For this review, take the finished solid that the model builds, in its own axes (mm). Face numbers are marked on the shaded views. A direction names the side the tool comes from. Coordinates: 2 decimals unless noted, no trailing zeros. Loops run counter-clockwise (first coordinate to the right, second up) from the corner with the lowest first, then second, coordinate; pieces in that order, holes last. Notation, with made-up numbers: (18, 39) -> (33, 39) arc R14 ccw to (33, 61) -> close; hole circle Ø3 at (29.25, 53). An arc over 180 degrees is marked (long way). Use a Markdown table: item, result.
from build123d import *
from build123d.topology import SkipClean

# Parameters (mm, degrees)
SKETCH1_W                 = 57.15
SKETCH1_H                 = 37.592
BOSS_EXTRUDE1_DEPTH       = 10.16
SKETCH2_W                 = 0.254
SKETCH2_H                 = 37.592
SKETCH2_W_2               = 2.032
BOSS_EXTRUDE2_DEPTH       = 2.54
SKETCH3_R                 = 6.35
CUT_EXTRUDE1_DEPTH        = 21.082
SKETCH4_R                 = 2.032
CUT_EXTRUDE2_DEPTH        = 5.08
SKETCH5_W                 = 2.54
SKETCH5_H                 = 0.254
BOSS_EXTRUDE3_DEPTH       = 3.048
MIRROR2_COPY_1_SKETCH_W   = 57.15
MIRROR2_COPY_1_SKETCH_H   = 37.592
MIRROR2_COPY_1_DEPTH      = 10.16
MIRROR2_COPY_2_SKETCH_W   = 0.254
MIRROR2_COPY_2_SKETCH_H   = 37.592
MIRROR2_COPY_2_SKETCH_W_2 = 2.032
MIRROR2_COPY_2_DEPTH      = 2.54
MIRROR2_COPY_3_SKETCH_R   = 6.35
MIRROR2_COPY_3_DEPTH      = 21.082
MIRROR2_COPY_4_SKETCH_R   = 2.032
MIRROR2_COPY_4_DEPTH      = 5.08
MIRROR2_COPY_5_SKETCH_W   = 2.54
MIRROR2_COPY_5_SKETCH_H   = 0.254
MIRROR2_COPY_5_DEPTH      = 3.048


with BuildPart() as part:
    # Sketch1 → Boss-Extrude1 (new body)
    with BuildSketch(Plane.XY):
        with Locations((0.47625, 18.796)):
            Rectangle(SKETCH1_W, SKETCH1_H)
    boss_extrude1 = extrude(amount=BOSS_EXTRUDE1_DEPTH)

    # Sketch2 → Boss-Extrude2 (add)
    with BuildSketch(Plane.XY.offset(10.16)):
        with Locations((-19.97075, 18.796)):
            Rectangle(SKETCH2_W, SKETCH2_H)
        with Locations((-18.57375, 18.796)):
            Rectangle(SKETCH2_W_2, SKETCH2_H)
        with Locations((-17.17675, 18.796)):
            Rectangle(SKETCH2_W, SKETCH2_H)
    boss_extrude2 = extrude(amount=BOSS_EXTRUDE2_DEPTH)

    # Sketch3 → Cut-Extrude1 (cut)
    with BuildSketch(Plane.XY.offset(10.16)):
        with Locations((-28.09875, 0)):
            Circle(SKETCH3_R)
    cut_extrude1 = extrude(amount=-CUT_EXTRUDE1_DEPTH, mode=Mode.SUBTRACT)

    # Sketch4 → Cut-Extrude2 (cut)
    with BuildSketch(Plane(origin=(0, 0, 0), x_dir=(-1, 0, 0), z_dir=(0, 0, -1))):
        with Locations((12.004431959, 16.094318041)):
            Circle(SKETCH4_R)
    cut_extrude2 = extrude(amount=-CUT_EXTRUDE2_DEPTH, mode=Mode.SUBTRACT)

    # Sketch5 → Boss-Extrude3 (add)
    with BuildSketch(Plane.ZY.offset(20.09775)):
        with Locations((11.43, 37.465)):
            Rectangle(SKETCH5_W, SKETCH5_H)
    boss_extrude3 = extrude(amount=-BOSS_EXTRUDE3_DEPTH)

    # Mirror1: Boss-Extrude1, Boss-Extrude2, Cut-Extrude1, Cut-Extrude2, Boss-Extrude3 across plane
    with SkipClean():  # the faces are left unmerged after this step: merging them gives an invalid solid
        add(boss_extrude1.mirror(Plane(origin=(-28.09875, 37.592, 10.16), x_dir=(0, 0, 1), z_dir=(1, 0, 0))))
        add(boss_extrude2.mirror(Plane(origin=(-28.09875, 37.592, 10.16), x_dir=(0, 0, 1), z_dir=(1, 0, 0))))
        add(cut_extrude1.mirror(Plane(origin=(-28.09875, 37.592, 10.16), x_dir=(0, 0, 1), z_dir=(1, 0, 0))), mode=Mode.SUBTRACT)
        add(cut_extrude2.mirror(Plane(origin=(-28.09875, 37.592, 10.16), x_dir=(0, 0, 1), z_dir=(1, 0, 0))), mode=Mode.SUBTRACT)
        add(boss_extrude3.mirror(Plane(origin=(-28.09875, 37.592, 10.16), x_dir=(0, 0, 1), z_dir=(1, 0, 0))))
    add(part.part.scale(1), mode=Mode.REPLACE)  # the faces are merged on a copy

    # Mirror2: Boss-Extrude1, Boss-Extrude2, Cut-Extrude1, Cut-Extrude2, Boss-Extrude3 across plane
    with SkipClean():  # the faces are left unmerged after this step: merging them gives an invalid solid
        add(boss_extrude1.mirror(Plane.ZX))
        add(boss_extrude2.mirror(Plane.ZX))
        add(cut_extrude1.mirror(Plane.ZX), mode=Mode.SUBTRACT)
        add(cut_extrude2.mirror(Plane.ZX), mode=Mode.SUBTRACT)
        add(boss_extrude3.mirror(Plane.ZX))
    add(part.part.scale(1), mode=Mode.REPLACE)  # the faces are merged on a copy

    # Mirror2 copy 1 sketch → Mirror2 copy 1 (add)
    with BuildSketch(Plane(origin=(-56.1975, 0, 0), x_dir=(-1, 0, 0), z_dir=(0, 0, 1))):
        with Locations((0.47625, 18.796)):
            Rectangle(MIRROR2_COPY_1_SKETCH_W, MIRROR2_COPY_1_SKETCH_H)
    extrude(amount=MIRROR2_COPY_1_DEPTH)

    # Mirror2 copy 2 sketch → Mirror2 copy 2 (add)
    with BuildSketch(Plane(origin=(-56.1975, 0, 10.16), x_dir=(-1, 0, 0), z_dir=(0, 0, 1))):
        with Locations((-19.97075, 18.796)):
            Rectangle(MIRROR2_COPY_2_SKETCH_W, MIRROR2_COPY_2_SKETCH_H)
        with Locations((-18.57375, 18.796)):
            Rectangle(MIRROR2_COPY_2_SKETCH_W_2, MIRROR2_COPY_2_SKETCH_H)
        with Locations((-17.17675, 18.796)):
            Rectangle(MIRROR2_COPY_2_SKETCH_W, MIRROR2_COPY_2_SKETCH_H)
    extrude(amount=MIRROR2_COPY_2_DEPTH)

    # Mirror2 copy 3 sketch → Mirror2 copy 3 (cut)
    with SkipClean():  # the faces are left unmerged after this step: merging them gives an invalid solid
        with BuildSketch(Plane(origin=(-56.1975, 0, 10.16), x_dir=(-1, 0, 0), z_dir=(0, 0, 1))):
            with Locations((-28.09875, 0)):
                Circle(MIRROR2_COPY_3_SKETCH_R)
        extrude(amount=-MIRROR2_COPY_3_DEPTH, mode=Mode.SUBTRACT)

    # Mirror2 copy 4 sketch → Mirror2 copy 4 (cut)
    with SkipClean():  # the faces are left unmerged after this step: merging them gives an invalid solid
        with BuildSketch(Plane(origin=(-56.1975, 0, 0), x_dir=(1, 0, 0), z_dir=(0, 0, -1))):
            with Locations((12.004431959, 16.094318041)):
                Circle(MIRROR2_COPY_4_SKETCH_R)
        extrude(amount=-MIRROR2_COPY_4_DEPTH, mode=Mode.SUBTRACT)

    # Mirror2 copy 5 sketch → Mirror2 copy 5 (add)
    with SkipClean():  # the faces are left unmerged after this step: merging them gives an invalid solid
        with BuildSketch(Plane(origin=(-36.09975, 0, 0), x_dir=(0, 0, 1), z_dir=(1, 0, 0))):
            with Locations((11.43, 37.465)):
                Rectangle(MIRROR2_COPY_5_SKETCH_W, MIRROR2_COPY_5_SKETCH_H)
        extrude(amount=-MIRROR2_COPY_5_DEPTH)


solid = part.part
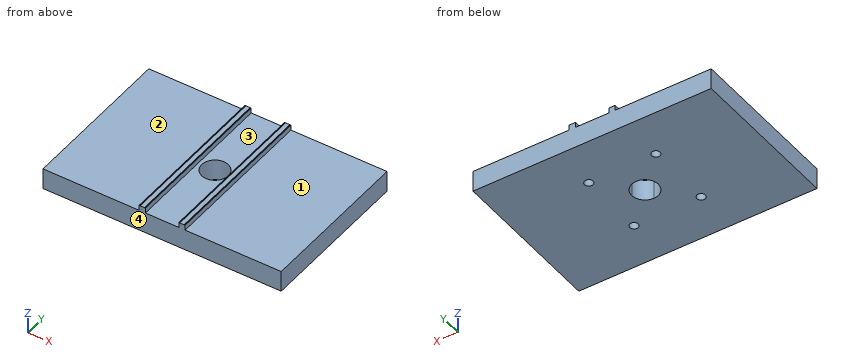
(1) Take a section at B-B on x = -29.5. Write out the cut boundary in (y, z), plus the area to 3 significant figures.
Found:
| item | result |
|---|---|
| outline | (-37.59, 0) -> (-6.19, 0) -> (-6.19, 10.16) -> (-37.59, 10.16) -> close; (6.19, 0) -> (37.59, 0) -> (37.59, 10.16) -> (6.19, 10.16) -> close |
| area | 638 mm^2 |
(2) Take a section at C-C on z = 3. Write out the cut boundary in (x, y), plus the area to 3 significant figures.
Found:
| item | result |
|---|---|
| outline | (-85.25, -37.59) -> (29.05, -37.59) -> (29.05, 37.59) -> (-85.25, 37.59) -> close; hole circle Ø4.06 at (-44.19, -16.09); hole circle Ø4.06 at (-44.19, 16.09); hole circle Ø12.7 at (-28.1, 0); hole circle Ø4.06 at (-12, -16.09); hole circle Ø4.06 at (-12, 16.09) |
| area | 8,410 mm^2 |
(3) For line 1 along X through (y, z) = (16, 2); line 2 along X through (y, z) = (0, 5); line 3 along X through (y, z) = (9, 11.5), list the stretches that pass through material, from the lowest coordinate up.
Found:
| item | result |
|---|---|
| line 1 | x = -85.25 to -46.22, -42.16 to -14.03, -9.97 to 29.05 |
| line 2 | x = -85.25 to -34.45, -21.75 to 29.05 |
| line 3 | x = -39.15 to -38.89, -38.64 to -36.61, -36.35 to -36.1, -20.1 to -19.84, -19.59 to -17.56, -17.3 to -17.05 |
(4) For pin 1 Ø3 at (y, z) = (-6, 12) entering from -X; pin 2 Ø23 at (x, y) = (-4, -11.5) entering from +Z; pin 3 Ø0.8 at (y, z) = (17, 11) entering from +X, all flat-tipped, find the tip position at first contact; note any pin that passes through.
Found:
| item | result |
|---|---|
| pin 1 | stops at x = -39.15 |
| pin 2 | stops at z = 10.16 |
| pin 3 | stops at x = -17.05 |
(5) Take a section at D-D on x = -44. Write out the cut boundary in (y, z), plus the area to 3 significant figures.
Found:
| item | result |
|---|---|
| outline | (-37.59, 0) -> (-18.12, 0) -> (-18.12, 5.08) -> (-14.07, 5.08) -> (-14.07, 0) -> (14.07, 0) -> (14.07, 5.08) -> (18.12, 5.08) -> (18.12, 0) -> (37.59, 0) -> (37.59, 10.16) -> (-37.59, 10.16) -> close |
| area | 723 mm^2 |
(6) Take a section at A-A on y = -30.5. Write out the cut boundary in (x, z).
Found:
| item | result |
|---|---|
| outline | (-85.25, 0) -> (29.05, 0) -> (29.05, 10.16) -> (-17.05, 10.16) -> (-17.05, 12.7) -> (-17.3, 12.7) -> (-17.3, 10.16) -> (-17.56, 10.16) -> (-17.56, 12.7) -> (-19.59, 12.7) -> (-19.59, 10.16) -> (-19.84, 10.16) -> (-19.84, 12.7) -> (-20.1, 12.7) -> (-20.1, 10.16) -> (-36.1, 10.16) -> (-36.1, 12.7) -> (-36.35, 12.7) -> (-36.35, 10.16) -> (-36.61, 10.16) -> (-36.61, 12.7) -> (-38.64, 12.7) -> (-38.64, 10.16) -> (-38.89, 10.16) -> (-38.89, 12.7) -> (-39.15, 12.7) -> (-39.15, 10.16) -> (-85.25, 10.16) -> close |
(7) For the marked faces 1, 2, 3 and 4, list the 3-axis set-ups (+Z, -Z, +X, -X, +Y, -Y) from which the entire face can be reached by the end or side of a thin tool; tool diameter is ignored.
Found:
| item | result |
|---|---|
| face 1 | +Z, +X, +Y, -Y |
| face 2 | +Z, -X, +Y, -Y |
| face 3 | +Z, +Y, -Y |
| face 4 | +Z, -Z, +X, -X, -Y |
